Here's how the part is built. I have some questions about the finished solid (model axes, mm). A direction names the side the tool comes from. Coordinates: 2 decimals unless noted, no trailing zeros. Order: outer loops, then holes, each group sorted by start corner. A loop starts at its lowest first (then second) coordinate and runs counter-clockwise, first axis right, second up. Notation, with made-up numbers: (54, 80) - (82, 80) arc R29 ccw to (82, 100) - close; hole circle Ø7 at (19, 53). An arc over 180 degrees is marked (long way). Answer in a Markdown table with one row per item. Add a question column.
Item 1: Thinking about a two-plate mould opening in Y: for faces 1 (the flat face through (-50, 4, 59)), 2 (the flat face through (26.04, 87.49, 24.9)), 3 (the flat face through (-0.2, 8.557, 79.3)), which applies, +Y half, -Y half, draft (parallel to the pull), parting line (faces both ways), or undercut?
Item 2: I want a section at C-C (x = 35.5). Please give me the cut outline in (y, z), plus the area to 3 significant figures.
Item 3: Will these pins go through, and if not, where does the flat tip stop? pin 1 Ø1.5 at (x, z) = (-15.5, 79.5) entering from +Y; pin 2 Ø0.6 at (y, z) = (8, 50.5) entering from +X; pin 3 Ø2 at (x, y) = (18, 5) entering from +Z.
Item 4: On a 3-axis mill with a long thin cutter (end or side, diameter ignored), from which of +Z, -Z, +X, -X, +Y, -Y can I reach the whole of each face in a straight line? I mean faces 4 (the flat face through (-48.9, 26.6, 57.2)), 5 (the flat face through (-1, 29, 80)). Say none if no direction works.
Item 5: If I drill on line 1 along Y through (x, z) = (14, 9); line 2 along Y through (x, z) = (-37.5, 67); line 3 along Z through (x, y) = (38.5, 17.5), over which ranges is the centre line in solid material (lowest first)? Write a range as from..to.
Item 6: I want a section at D-D (y = 56.5). Please give me the cut outline in (x, z).
```python
from build123d import *

# Parameters (mm, degrees)
BOSS_EXTRUDE2_DEPTH   = 80
CUT_EXTRUDE6_DEPTH    = 80
FILLET4_R             = 8
FILLET6_R             = 8
BOSS_EXTRUDE3_DEPTH   = 5
CUT_EXTRUDE7_DEPTH    = 53
SKETCH8_W             = 0.862104353
SKETCH8_H             = 1.284661266
CUT_EXTRUDE8_DEPTH    = 53
SKETCH9_R             = 2.6
CUT_EXTRUDE9_DEPTH    = 53
CHAMFER1_SIZE         = 2
CHAMFER1_SIZE2        = 0.352653961
CHAMFER2_SIZE         = 2
CHAMFER2_SIZE2        = 1.125418904
CHAMFER2_PART_2_SIZE  = 2
CHAMFER2_PART_2_SIZE2 = 1.486326178
CHAMFER2_PART_3_SIZE  = 2
CHAMFER2_PART_3_SIZE2 = 12.979996821
FILLET7_R             = 3


with BuildPart() as part:
    # Sketch4 → Boss-Extrude2 (new body)
    with BuildSketch(Plane.XY):
        Polygon((0, 90), (25, 90), (27.110033345, 84.90483075), (42.705570979, 33.625818377), (47.850101428, 30.956311994), (50, 22.038522927), (51.568309777, 22.038522927), (51.568309777, 20.486613591), (50, 20.486613591), (50, 19.211830923), (51.568309777, 19.211830923), (51.568309777, 17.666105021), (50, 17.666105021), (47.850101428, 8.556688769), (39.441409504, 8.556688769), (39.441409504, 7.272027503), (50, 7.272027503), (50, 0), (0, 0), align=None)
    extrude(amount=BOSS_EXTRUDE2_DEPTH)

    # Sketch5 → Cut-Extrude6 (cut)
    with BuildSketch(Plane.ZY):
        Polygon((80, 90), (45.569058945, 90), (57.70788513, 75.886568849), (65.410192712, 42.801872405), (80, 37.57441702), align=None)
        Polygon((30, 72.649548533), (0, 72.649548533), (0, 0), (38.690390773, 0), align=None)
    extrude(amount=-CUT_EXTRUDE6_DEPTH, mode=Mode.SUBTRACT)

    # Fillet4
    fillet4_edges = [part.edges().sort_by_distance(p)[0] for p in [
        (15.418622329, 72.649548533, 0),
        (15.418622329, 72.649548533, 30),
    ]]
    fillet(fillet4_edges, radius=FILLET4_R)

    # Fillet6
    fillet6_edges = [part.edges().sort_by_distance(p)[0] for p in [
        (12.5, 90, 0),
        (12.5, 90, 45.569058945),
    ]]
    fillet(fillet6_edges, radius=FILLET6_R)

    # Sketch6 → Boss-Extrude3 (add)
    with BuildSketch(Plane.XY.offset(80)):
        Polygon((51.568309777, 22.038522927), (50, 22.038522927), (0, 22.038522927), (0, 20.486613591), (50, 20.486613591), (51.568309777, 20.486613591), align=None)
        Polygon((50, 19.211830923), (0, 19.211830923), (0, 17.666105021), (50, 17.666105021), (51.568309777, 17.666105021), (51.568309777, 19.211830923), align=None)
    extrude(amount=BOSS_EXTRUDE3_DEPTH)

    # Sketch7 → Cut-Extrude7 (cut)
    with BuildSketch(Plane.ZY):
        Polygon((80, 17.666105021), (78.657986015, 9.613389648), (80, 9.613389648), align=None)
    extrude(amount=-CUT_EXTRUDE7_DEPTH, mode=Mode.SUBTRACT)

    # Sketch8 → Cut-Extrude8 (cut)
    with BuildSketch(Plane(origin=(39.441409504, 0, 0), x_dir=(0, 0, -1), z_dir=(1, 0, 0))):
        with Locations((-79.568947823, 7.914358136)):
            Rectangle(SKETCH8_W, SKETCH8_H)
    extrude(amount=-CUT_EXTRUDE8_DEPTH, mode=Mode.SUBTRACT)

    # Sketch9 → Cut-Extrude9 (cut)
    with BuildSketch(Plane.XZ.offset(-72.649548533)):
        with Locations((0, 15.44996627)):
            Circle(SKETCH9_R)
    extrude(amount=-CUT_EXTRUDE9_DEPTH, mode=Mode.SUBTRACT)

    # Chamfer1
    chamfer1_edges = [part.edges().sort_by_distance(p)[0] for p in [
        (2.6, 72.649548533, 15.44996627),
    ]]
    chamfer1_side = [part.faces().sort_by_distance(p)[0] for p in [
        (15.75727698, 72.649548533, 15.44996627),
    ]]
    chamfer(chamfer1_edges, length=CHAMFER1_SIZE, length2=CHAMFER1_SIZE2, reference=chamfer1_side[0])

    # Chamfer2
    chamfer2_edges = [part.edges().sort_by_distance(p)[0] for p in [
        (20.75233985, 37.57441702, 80),
    ]]
    chamfer2_side = [part.faces().sort_by_distance(p)[0] for p in [
        (23.38094375, 29.531291641, 80),
    ]]
    chamfer(chamfer2_edges, length=CHAMFER2_SIZE, length2=CHAMFER2_SIZE2, reference=chamfer2_side[0])

    # Chamfer2 part 2
    chamfer2_part_2_edges = [part.edges().sort_by_distance(p)[0] for p in [
        (19.957424217, 42.801872405, 65.410192712),
    ]]
    chamfer2_part_2_side = [part.faces().sort_by_distance(p)[0] for p in [
        (17.56283553, 58.548959268, 61.744180339),
    ]]
    chamfer(chamfer2_part_2_edges, length=CHAMFER2_PART_2_SIZE, length2=CHAMFER2_PART_2_SIZE2, reference=chamfer2_part_2_side[0])

    # Chamfer2 part 3
    chamfer2_part_3_edges = [part.edges().sort_by_distance(p)[0] for p in [
        (14.926383206, 75.886568849, 57.70788513),
    ]]
    chamfer2_part_3_side = [part.faces().sort_by_distance(p)[0] for p in [
        (14.071000693, 81.431316149, 52.938901387),
    ]]
    chamfer(chamfer2_part_3_edges, length=CHAMFER2_PART_3_SIZE, length2=CHAMFER2_PART_3_SIZE2, reference=chamfer2_part_3_side[0])

    # Fillet7
    fillet7_edges = [part.edges().sort_by_distance(p)[0] for p in [
        (19.661214366, 44.749781992, 64.956708159),
        (20.694615521, 37.954018761, 78.940533046),
        (20.033659992, 42.3005373, 66.809417005),
        (21.056470857, 35.57441702, 80),
    ]]
    fillet(fillet7_edges, radius=FILLET7_R)

    # Mirror2: part across plane


with BuildPart() as part_1:
    add(part.part)
    add(part.part.mirror(Plane(origin=(0, 90, 80), x_dir=(0, 0, 1), z_dir=(1, 0, 0))))


solid = part_1.part
```
Values follow:
| question | item | result |
|---|---|---|
| 1 | face 1 | draft |
| 1 | face 2 | +Y half |
| 1 | face 3 | undercut |
| 2 | outline | (0, 38.69) - (57.32, 31.83) - (57.32, 62.03) - (45.37, 64.81) arc R3 cw to (44.24, 65.34) - (43.01, 66.27) arc R3 cw to (42, 67.65) - (38.39, 77.73) arc R3 ccw to (36.78, 79.46) - (36.16, 79.74) arc R3 ccw to (34.94, 80) - (22.04, 80) - (22.04, 85) - (20.49, 85) - (20.49, 80) - (19.21, 80) - (19.21, 85) - (17.67, 85) - (17.67, 80) - (9.61, 78.66) - (9.61, 80) - (8.56, 80) - (8.56, 79.14) - (7.27, 79.14) - (7.27, 80) - (0, 80) - close |
| 2 | area | 2,300 mm^2 |
| 3 | pin 1 | stops at y = 37.77 |
| 3 | pin 2 | stops at x = 39.44 |
| 3 | pin 3 | stops at z = 80 |
| 4 | face 4 | +Z, -Z, -X, +Y |
| 4 | face 5 | +Z, +X, -X, +Y |
| 5 | line 1 | y = 72.65..90 |
| 5 | line 2 | y = 0..42.33 |
| 5 | line 3 | z = 36.6..79.97 |
| 6 | outline | (-35.75, 31.93) - (35.75, 31.93) - (35.75, 62.22) - (-35.75, 62.22) - close |
